For this review, take the finished solid that the model builds, in its own axes (mm). A direction names the side the tool comes from. Round coordinates to 2 decimals unless told otherwise and drop trailing zeros. Write each loop counter-clockwise with the first axis right and the second up, starting at its lowest first coordinate (ties: lowest second). Pieces come first, ordered by that corner, then holes. Notation, with made-up numbers: (35.25, -35.5) -> (55.25, -35.5) arc R28 cw to (55.25, -15.5) -> close; hole circle Ø3 at (35.25, 76). An arc over 180 degrees is marked (long way). Answer in a Markdown table with one row per item.
Autodesk Inventor part; units mm, degrees
ref_plane "YZ Plane" through (0, 0, 0) normal (1, 0, 0) x (0, 1, 0)
ref_plane "XZ Plane" through (0, 0, 0) normal (0, 1, 0) x (-1, 0, 0)
ref_plane "XY Plane" through (0, 0, 0) normal (0, 0, 1) x (1, 0, 0)
sketch "Sketch1" plane through (0, 0, 0) normal (0, 0, 1) x (1, 0, 0)
  circle A0 centre (0, 0) radius 14.7
  dimension "d0" = 29.4
extrude "Extrusion1" add sketch "Sketch1" along normal blind 14
sketch "Sketch2" plane through (0, 0, 14) normal (0, 0, 1) x (1, 0, 0)
  circle A0 centre (0, 0) radius 11.2
  dimension "d3" = 22.4
extrude "Extrusion2" add sketch "Sketch2" along normal blind 4
fillet "Fillet1" radius 3.2 1 edges at (-14.7, 0, 14)
fillet "Fillet2" radius 4 1 edges at (-11.2, 0, 18)
sketch "Sketch3" plane through (0, 0, 0) normal (1, 0, 0) x (0, 1, 0)
  line L0 (-7.2, 18) -> (7.2, 18)
  line L1 (7.2, 18) -> (-7.2, 18)
  arc A0 (7, 18) -> (-7, 18) centre (0, 11.3333) ccw
  line L2 (0, 18) -> (0, 21)
  point P0 (0, 0)
  dimension "d9" = 14
revolve "Revolution1" add sketch "Sketch3" angle 360 about axis through (0, 0, 18) along (0, 0, 1) picked at (4.1722, 18.4238) contours L2 A0 L0
sketch "Sketch4" plane through (0, 0, 0) normal (0, 0, -1) x (-1, 0, 0)
  arc A0 (-1.7555, -20.7411) -> (1.7555, -20.7411) centre (0, -18.9612) ccw
  line L0 (1.7555, -20.7411) -> (11.2352, -11.3917)
  line L1 (-1.7555, -20.7411) -> (-11.2549, -11.3723)
  arc A1 (1.7361, 20.7603) -> (-1.7554, 20.7412) centre (0.0001, 18.9613) ccw
  line L2 (1.7361, 20.7603) -> (11.2352, 11.3917)
  line L3 (-1.7554, 20.7412) -> (-11.2549, 11.3723)
  arc A2 (-11.2352, 11.3917) -> (-11.2352, -11.3917) centre (0, 0) ccw
  arc A3 (11.2352, -11.3917) -> (11.2352, 11.3917) centre (0, 0) ccw
  circle A4 centre (0, 18) radius 1.5
  circle A5 centre (0, -18) radius 1.5
  dimension "d13" = 5
  dimension "d19" = 32
  dimension "d22" = 3
  dimension "d23" = 3
sketch "Sketch5" plane through (0, 0, 0) normal (0, 1, 0) x (-1, 0, 0)
  point P0 (0, 0)
extrude "Extrusion4" add sketch "Sketch4" along normal blind 1
fillet "Fillet5" radius 1 1 edges at (-14.7, 0, 0)
sketch "Sketch7" plane through (0, 0, -1) normal (0, 0, -1) x (-1, 0, 0)
  line L0 (-11.2352, -11.3917) -> (-1.7555, -20.7411)
  line L1 (1.7555, -20.7411) -> (11.2352, -11.3917)
  arc A0 (-1.7555, -20.7411) -> (1.7555, -20.7411) centre (0, -18.9612) ccw
  arc A1 (-11.2352, 11.3917) -> (-11.2352, -11.3917) centre (0, 0) ccw
  line L2 (-1.7554, 20.7412) -> (-11.2352, 11.3917)
  line L3 (11.2352, 11.3917) -> (1.7361, 20.7603)
  circle A2 centre (0, -18) radius 1.5
  circle A3 centre (0, 18) radius 1.5
  arc A4 (-1.7555, -20.7411) -> (1.7555, -20.7411) centre (0, -18.9612) ccw
  line L4 (1.7555, -20.7411) -> (11.2352, -11.3917)
  arc A5 (11.2352, -11.3917) -> (11.2352, 11.3917) centre (0, 0) ccw
  line L5 (11.2352, 11.3917) -> (1.7361, 20.7603)
  arc A6 (1.7361, 20.7603) -> (-1.7554, 20.7412) centre (0.0001, 18.9613) ccw
  line L6 (-1.7554, 20.7412) -> (-11.2352, 11.3917)
  arc A7 (-11.2352, 11.3917) -> (-11.2352, -11.3917) centre (0, 0) ccw
  line L7 (-11.2352, -11.3917) -> (-1.7555, -20.7411)
  arc A8 (1.7361, 20.7603) -> (-1.7554, 20.7412) centre (0.0001, 18.9613) ccw
  arc A9 (11.9374, -12.1037) -> (11.9374, 12.1037) centre (0, 0) ccw
  line L8 (11.9374, -12.1037) -> (2.4577, -21.4531)
  arc A10 (-2.4577, -21.4531) -> (2.4577, -21.4531) centre (0, -18.9612) ccw
  line L9 (-2.4577, -21.4531) -> (-11.9374, -12.1037)
  arc A11 (-11.9374, 12.1037) -> (-11.9374, -12.1037) centre (0, 0) ccw
  line L10 (-11.9374, 12.1037) -> (-2.4576, 21.4532)
  arc A12 (2.4347, 21.4758) -> (-2.4576, 21.4532) centre (0.0001, 18.9613) ccw
  line L11 (2.4347, 21.4758) -> (11.9374, 12.1037)
  dimension "d27" = 1
extrude "Extrusion5" add sketch "Sketch7" along normal blind 2 contours A1 L2 A6 L3 A5 L1 A0 L0 | L8 A10 L9 A11 L10 A12 L11 A9
properties part number "wheel2"
1) Clearance check with flat-ended pins moving along their axes: pin 1 Ø12 at (x, y) = (-10.5, 17) entering from +Z; pin 2 Ø5 at (x, z) = (-1.5, 17.5) entering from +Y; pin 3 Ø4 at (x, y) = (0, -18) entering from +Z; pin 4 Ø11.5 at (x, y) = (3.5, 1) entering from +Z. State where each tip first meets the part, or that it passes through.
Solved:
| item | result |
|---|---|
| pin 1 | z = 12.82 |
| pin 2 | y = 11.02 |
| pin 3 | z = 0 |
| pin 4 | z = 21 |
2) Mouldability with a two-part tool opening along X and no side actions: class faces 1 (the flat face through (7.131, -16.844, -1.986)), 2 (the cylindrical face through (-0.03, -21.46, -0.49)), 3 (the cylindrical face through (0.195, -19.487, -1.479)) as pulls with the +X half, pulls with the -X half, needs draft (parallel to the pull), parting line crosses it, or undercut.
Solved:
| item | result |
|---|---|
| face 1 | pulls with the +X half |
| face 2 | parting line crosses it |
| face 3 | undercut |
3) Consider section A-A on y = -18. State the section outline as (x, z) points, then the cut area to 3 significant figures.
Solved:
| item | result |
|---|---|
| outline | (-5.96, -3) -> (-1.5, -3) -> (-1.5, 0) -> (-4.53, 0) -> (-4.53, -1) -> (-5.96, -1) -> close; (1.5, -3) -> (5.96, -3) -> (5.96, -1) -> (4.53, -1) -> (4.53, 0) -> (1.5, 0) -> close |
| area | 23.9 mm² |
4) For faces 4 (the cylindrical face through (0.04, 21.46, -0.49)), 5 (the flat face through (-6.43, -16.13, -0.49)), 6 (the flat face through (13, 10, -1)), list the 3-axis set-ups (+Z, -Z, +X, -X, +Y, -Y) from which the entire face can be reached by the end or side of a thin tool; tool diameter is ignored.
Solved:
| item | result |
|---|---|
| face 4 | +Z, +Y |
| face 5 | +Z, -X, -Y |
| face 6 | +Z |
5) Consider section D-D on z = 5.75. State the section outline as (x, y) points.
Solved:
| item | result |
|---|---|
| outline | circle Ø29.4 at (0, 0) |
6) For line 1 (Z direction, x = 5, y = -15); line 2 (Z direction, x = -5, y = 5.5); line 3 (Y direction, x = 5, z = 13.25), list the stretches that pass through material, from the lowest coordinate up. Write a range as [from, to].
Solved:
| item | result |
|---|---|
| line 1 | [-3, 0] |
| line 2 | [-3, 17.99] |
| line 3 | [-12.6, 12.6] |
7) Consider section B-B on z = -0.5. State the section outline as (x, y) points.
Solved:
| item | result |
|---|---|
| outline | (-11.24, -11.39) -> (-1.76, -20.74) arc R2.5 ccw to (1.76, -20.74) -> (11.25, -11.37) arc R16 ccw to (11.25, 11.37) -> (1.76, 20.74) arc R2.5 ccw to (-1.74, 20.76) -> (-11.24, 11.39) arc R16 ccw to start; hole circle Ø3 at (0, -18); hole circle Ø3 at (0, 18) |
